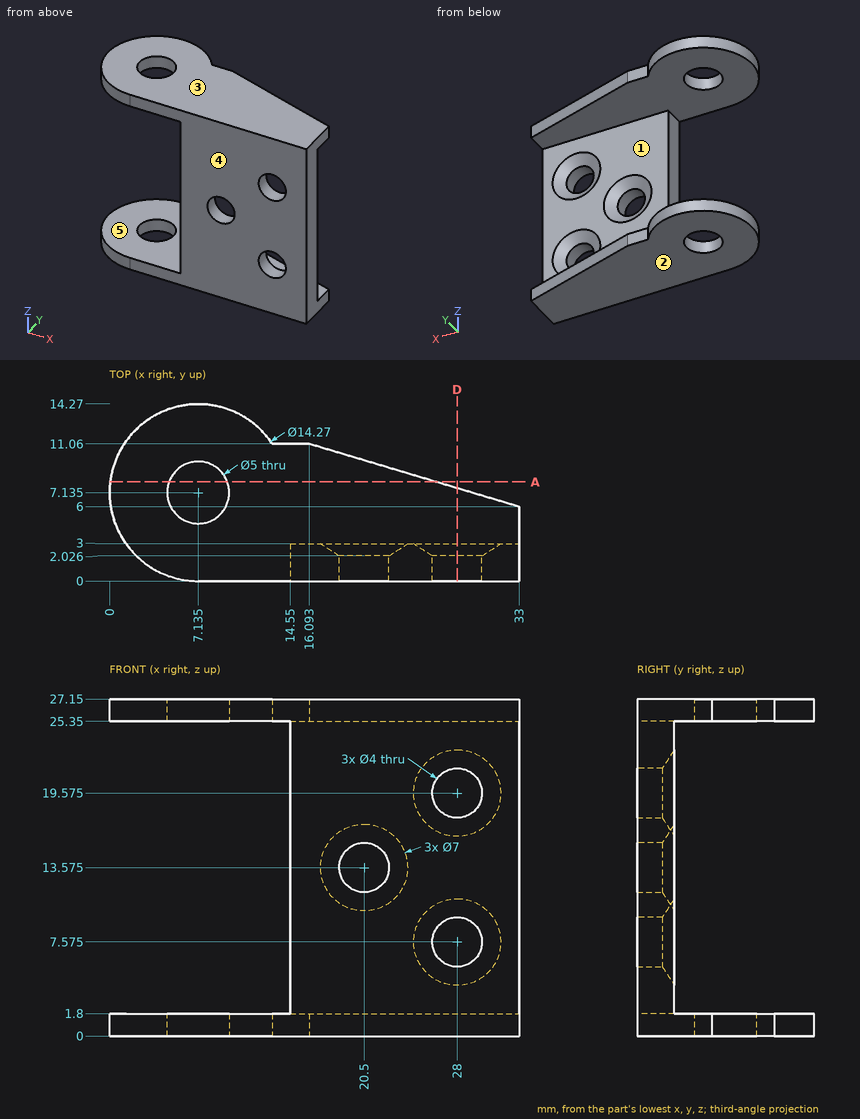
For this review, use the dimensioned drawing (mm, ordinates from the lowest corner) and the shaded views. A direction names the side the tool comes from. Round coordinates to 2 decimals unless told otherwise and drop trailing zeros. Write each loop counter-clockwise with the first axis right and the second up, starting at its lowest first coordinate (ties: lowest second). Pieces come first, ordered by that corner, then holes. Notation, with made-up numbers: M -25,29 L -11,29 A20 ccw -11,45 Z; hole C 55.5,57 d7. An arc over 180 degrees is marked long. Write item = value, one per line. Start each with the question number.
(1) Clearance check with flat-ended pins moving along their axes: pin 1 Ø6 at (x, y) = (7.135, 7.135) entering from -Z; pin 2 Ø1 at (x, z) = (15, 15.5) entering from +Y; pin 3 Ø2.5 at (y, z) = (2, 8) entering from -X; pin 4 Ø1.4 at (x, z) = (14, 1) entering from +Y. State where each tip first meets the part, or that it passes through.
(2) The part is to be moulded in two halves that separate along Z. For the marked faces 1, 2 and 3, say which applies: +Z half, -Z half, draft (parallel to the pull), parting line (faces both ways), or undercut.
(3) For the marked faces 4 and 5, list the 3-axis set-ups (+Z, -Z, +X, -X, +Y, -Y) from which the entire face can be reached by the end or side of a thin tool; tool diameter is ignored.
(4) We need section D-D (x = 28). Give the number of separate pieces and of enclosed holes in the cut face.
(5) We need section A-A (y = 8). Give the boundary of the cut face in (x, z).
(6) For line 1 along Z through (x, y) = (2.5, 4.5); line 2 along X through (y, z) = (2, 16.75); line 3 along Y through (x, z) = (24.5, 11.75), list the stretches that pass through material, from the lowest coordinate up.
Results found:
q1.pin_1 = 0
q1.pin_2 = 3
q1.pin_3 = 14.55
q1.pin_4 = 11.06
q2.face_1 = undercut
q2.face_2 = -Z half
q2.face_3 = +Z half
q3.face_4 = +Z, -Z, +X, -X, -Y
q3.face_5 = -X, +Y
q4.separate_pieces = 3
q4.enclosed_holes = 0
q5.outline = M 0.05,0 L 4.79,0 L 4.79,1.8 L 0.05,1.8 Z; M 0.05,25.35 L 4.79,25.35 L 4.79,27.15 L 0.05,27.15 Z; M 9.48,0 L 26.32,0 L 26.32,1.8 L 9.48,1.8 Z; M 9.48,25.35 L 26.32,25.35 L 26.32,27.15 L 9.48,27.15 Z
q6.line_1 = 0 to 1.8, 25.35 to 27.15
q6.line_2 = 14.55 to 33
q6.line_3 = 0 to 3
